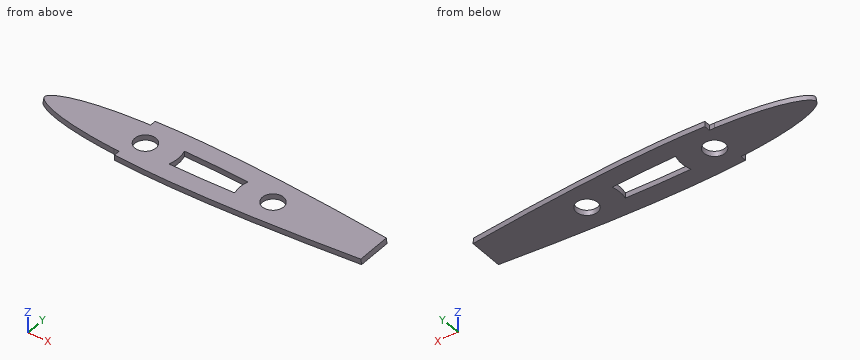
```python
from build123d import *

# Parameters (mm, degrees)
BOSS_EXTRUDE1_DEPTH     = 3.175
SKETCH2_R               = 6.35
CUT_EXTRUDE1_DEPTH      = 3.175
CUT_EXTRUDE2_DEPTH      = 17.98531302
CUT_EXTRUDE2_DEPTH_BACK = 17.98531302
CUT_EXTRUDE3_DEPTH      = 7.62


with BuildPart() as part:
    # Sketch1 → Boss-Extrude1 (new body)
    with BuildSketch(Plane.XY):
        with BuildLine():
            add(Edge.make_bspline(
                [(283.0068, 0.356588568), (282.901747419, 0.44462405), (282.222988768, 0.361501496), (281.014292834, 0.701750535), (278.797705315, 0.912055534), (275.811625252, 1.363395917), (271.96510687, 1.867061556), (267.326448481, 2.487806401), (261.907718596, 3.189499382), (255.748156548, 3.970743632), (248.883761402, 4.817852882), (241.357474346, 5.719362844), (233.215556988, 6.664092103), (224.508147533, 7.639178426), (215.288960535, 8.632716794), (205.614900546, 9.632367333), (195.545587828, 10.625227013), (185.143130495, 11.597359066), (174.471591387, 12.536001404), (163.596880752, 13.425461607), (152.585818931, 14.251236992), (141.506392817, 14.997996378), (130.426867175, 15.650125673), (119.415450083, 16.19114965), (108.540147703, 16.606641404), (97.867696152, 16.883046032), (87.464049003, 17.006862886), (77.393132365, 16.968265808), (67.717036062, 16.75979946), (58.495320886, 16.376179449), (49.784748261, 15.816402284), (41.638853683, 15.082152298), (34.107484228, 14.179164014), (27.236546007, 13.115120527), (21.067675242, 11.901134861), (15.637028536, 10.550933877), (10.975465177, 9.077683717), (7.106668967, 7.49510566), (4.042977604, 5.813906592), (1.789105378, 4.030768344), (0.345518556, 2.10255275), (-0.161023932, 0), (0.345518556, -2.10255275), (1.789105378, -4.030768344), (4.042977604, -5.813906592), (7.106668967, -7.49510566), (10.975465177, -9.077683717), (15.637028536, -10.550933877), (21.067675242, -11.901134861), (27.236546007, -13.115120527), (34.107484228, -14.179164014), (41.638853683, -15.082152298), (49.784748261, -15.816402284), (58.495320886, -16.376179449), (67.717036062, -16.75979946), (77.393132365, -16.968265808), (87.464049003, -17.006862886), (97.867696152, -16.883046032), (108.540147703, -16.606641404), (119.415450083, -16.19114965), (130.426867175, -15.650125673), (141.506392817, -14.997996378), (152.585818931, -14.251236992), (163.596880752, -13.425461607), (174.471591387, -12.536001404), (185.143130495, -11.597359066), (195.545587828, -10.625227013), (205.614900546, -9.632367333), (215.288960535, -8.632716794), (224.508147533, -7.639178426), (233.215556988, -6.664092103), (241.357474346, -5.719362844), (248.883761402, -4.817852882), (255.748156548, -3.970743632), (261.907718596, -3.189499382), (267.326448481, -2.487806401), (271.96510687, -1.867061556), (275.811625252, -1.363395917), (278.797705315, -0.912055534), (281.014292834, -0.701750535), (282.222988768, -0.361501496), (283.176929529, -0.478323569), (283.176929529, 0.214017725), (283.0068, 0.356588568)],
                knots=[0, 0, 0, 0, 0.000762215, 0.003044706, 0.006832246, 0.012101176, 0.018817536, 0.026939455, 0.036414848, 0.047184628, 0.059180413, 0.072327874, 0.086544061, 0.10174058, 0.117823336, 0.134691452, 0.152240154, 0.17036129, 0.188941008, 0.207865435, 0.227016078, 0.246275696, 0.265524943, 0.284644966, 0.303520118, 0.322034575, 0.340078353, 0.357542593, 0.374325482, 0.390329891, 0.40546389, 0.419643801, 0.432793371, 0.444843817, 0.455737921, 0.465428653, 0.47388632, 0.481101634, 0.487101684, 0.491975368, 0.495930678, 0.499382808, 0.502834938, 0.506790248, 0.511663932, 0.517663982, 0.524879296, 0.533336963, 0.543027695, 0.553921799, 0.565972245, 0.579121815, 0.593301726, 0.608435725, 0.624440134, 0.641223023, 0.658687263, 0.676731041, 0.695245498, 0.71412065, 0.733240673, 0.75248992, 0.771749538, 0.790900181, 0.809824608, 0.828404326, 0.846525462, 0.864074164, 0.88094228, 0.897025036, 0.912221555, 0.926437743, 0.939585203, 0.951580988, 0.962350768, 0.971826162, 0.979948081, 0.986664441, 0.991933371, 0.99572091, 0.998003402, 0.998765616, 1, 1, 1, 1], degree=3))
        make_face()
    extrude(amount=BOSS_EXTRUDE1_DEPTH)

    # Sketch2 → Cut-Extrude1 (cut)
    with BuildSketch(Plane.XY.offset(3.175)):
        with Locations((63.5, 0)):
            Circle(SKETCH2_R)
        with Locations((139.7, 0)):
            Circle(SKETCH2_R)
    extrude(amount=-CUT_EXTRUDE1_DEPTH, mode=Mode.SUBTRACT)

    # Sketch3 → Cut-Extrude2 (cut, two sides)
    with BuildSketch(Plane(origin=(0, 0, 0), x_dir=(1, 0, 0), z_dir=(0, 1, 0))) as cut_extrude2_sk:
        Polygon((280.502264678, 570.685147201), (200.220132014, 0), (199.773483328, -3.175), (283.134397147, -3.175), (283.134397147, 0), (283.134397147, 576.304397051), (-760.640477334, 1065.222635252), (-763.272609802, 1059.603385401), align=None)
    extrude(amount=CUT_EXTRUDE2_DEPTH, mode=Mode.SUBTRACT)
    extrude(cut_extrude2_sk.sketch, amount=-CUT_EXTRUDE2_DEPTH_BACK, mode=Mode.SUBTRACT)

    # Sketch5 → Cut-Loft1 section 0
    with BuildSketch(Plane.XY.offset(3.175)):
        with BuildLine():
            Line((57.15, -15.840717611), (57.15, -12.517848774))
            Line((57.15, -12.517848774), (54.102, -12.517848774))
            add(Edge.make_bspline(
                [(54.102, 12.517848774), (52.905073826, 12.446922239), (50.510877245, 12.29292233), (46.923042309, 12.02249839), (43.342906141, 11.709637993), (39.772343425, 11.350207554), (36.212958119, 10.940125109), (32.668672918, 10.473083309), (29.140579279, 9.942416236), (26.221744689, 9.439792705), (23.899631399, 8.996334016), (22.168124881, 8.641223297), (20.447130555, 8.261260302), (18.73921392, 7.85440932), (17.04583843, 7.418483842), (15.37131979, 6.950314461), (13.720374707, 6.446953018), (12.099093951, 5.903590986), (10.516736009, 5.316840777), (8.982942702, 4.676356823), (7.515425701, 3.975597981), (6.148367378, 3.214391725), (5.132435214, 2.525362189), (4.436328841, 1.942644965), (3.99449908, 1.50088383), (3.639558845, 1.055711416), (3.418173473, 0.67028204), (3.294529971, 0.303832168), (3.258254336, 8.98e-07), (3.294531501, -0.303834398), (3.41817022, -0.670279004), (3.63956519, -1.05571658), (3.994486701, -1.500874192), (4.436322379, -1.942640233), (5.13276687, -2.525613649), (6.148175252, -3.21424607), (7.515525046, -3.97567324), (8.982885795, -4.676313816), (10.516775422, -5.316870372), (12.099068229, -5.90357211), (13.720394844, -6.446967156), (15.371289631, -6.95029465), (17.045828606, -7.418477981), (18.739219111, -7.854412516), (20.44713727, -8.261264475), (22.168119663, -8.641219802), (23.899622625, -8.996332253), (26.221845214, -9.439810116), (29.140506404, -9.942404258), (32.668709943, -10.473088914), (36.212941173, -10.940123046), (39.772346311, -11.350206942), (43.342914131, -11.709640819), (46.923012021, -12.0224901), (50.510859023, -12.292917903), (52.905073826, -12.446922239), (54.102, -12.517848774)],
                knots=[0, 0, 0, 0, 0.03125, 0.0625, 0.09375, 0.125, 0.15625, 0.1875, 0.21875, 0.25, 0.265625, 0.28125, 0.296875, 0.3125, 0.328125, 0.34375, 0.359375, 0.375, 0.390625, 0.40625, 0.421875, 0.4375, 0.453125, 0.4609375, 0.46875, 0.4765625, 0.484375, 0.4921875, 0.5, 0.5078125, 0.515625, 0.5234375, 0.53125, 0.5390625, 0.546875, 0.5625, 0.578125, 0.59375, 0.609375, 0.625, 0.640625, 0.65625, 0.671875, 0.6875, 0.703125, 0.71875, 0.734375, 0.75, 0.78125, 0.8125, 0.84375, 0.875, 0.90625, 0.9375, 0.96875, 1, 1, 1, 1], degree=3))
            Line((54.102, 12.517848774), (57.15, 12.517848774))
            Line((57.15, 12.517848774), (57.15, 15.840717611))
            Line((57.15, 15.840717611), (57.15, 24.528656823))
            Line((57.15, 24.528656823), (-13.660315185, 32.196838039))
            Line((-13.660315185, 32.196838039), (4.751362513, -35.926369443))
            Line((4.751362513, -35.926369443), (57.15, -29.012871964))
            Line((57.15, -29.012871964), (57.15, -15.840717611))
        make_face()
    # Sketch4 → Cut-Loft1 section 1
    with BuildSketch(Plane(origin=(0, 0, 0), x_dir=(-1, 0, 0), z_dir=(0, 0, -1))):
        with BuildLine():
            Line((-57.15, -15.931097341), (-57.15, -12.614401813))
            Line((-57.15, -12.614401813), (-54.102, -12.614401813))
            add(Edge.make_bspline(
                [(-54.102, 12.614401813), (-52.892966304, 12.543650374), (-50.474562395, 12.389900929), (-46.850429349, 12.119518431), (-43.233994008, 11.80632974), (-39.627106768, 11.446155851), (-36.031309682, 11.034861155), (-32.450571185, 10.566087473), (-28.885974607, 10.033109549), (-25.936699002, 9.527992325), (-23.590171059, 9.082138578), (-21.840349809, 8.725010585), (-20.101018277, 8.342781179), (-18.374759552, 7.933393598), (-16.663038707, 7.494638099), (-14.970151675, 7.023265253), (-13.3008012, 6.516250081), (-11.661107617, 5.968693544), (-10.06037111, 5.377118947), (-8.508330893, 4.731019213), (-7.022897298, 4.023737888), (-5.63853584, 3.25470078), (-4.609088563, 2.55765795), (-3.903506054, 1.967798123), (-3.455598612, 1.52050909), (-3.095749955, 1.069692125), (-2.871302388, 0.679325256), (-2.745924545, 0.30796261), (-2.7091298, 9.1e-07), (-2.745926097, -0.307964873), (-2.871299087, -0.679322175), (-3.095756394, -1.069697364), (-3.455586055, -1.520499314), (-3.903499495, -1.967793321), (-4.609425021, -2.557913052), (-5.638340949, -3.254553026), (-7.022998045, -4.023814214), (-8.50827323, -4.730975626), (-10.060410962, -5.377148887), (-11.661081805, -5.968674575), (-13.300821123, -6.516264103), (-14.970122445, -7.02324602), (-16.6630295, -7.494632633), (-18.374764393, -7.933396571), (-20.10102481, -8.342785237), (-21.840344745, -8.725007186), (-23.590162295, -9.082136874), (-25.936800786, -9.528009858), (-28.88590077, -10.033097475), (-32.450608778, -10.56609314), (-36.031292313, -11.034859029), (-39.627110143, -11.446155342), (-43.234001329, -11.806332406), (-46.850400529, -12.119510514), (-50.474544843, -12.389896679), (-52.892966304, -12.543650374), (-54.102, -12.614401813)],
                knots=[0, 0, 0, 0, 0.03125, 0.0625, 0.09375, 0.125, 0.15625, 0.1875, 0.21875, 0.25, 0.265625, 0.28125, 0.296875, 0.3125, 0.328125, 0.34375, 0.359375, 0.375, 0.390625, 0.40625, 0.421875, 0.4375, 0.453125, 0.4609375, 0.46875, 0.4765625, 0.484375, 0.4921875, 0.5, 0.5078125, 0.515625, 0.5234375, 0.53125, 0.5390625, 0.546875, 0.5625, 0.578125, 0.59375, 0.609375, 0.625, 0.640625, 0.65625, 0.671875, 0.6875, 0.703125, 0.71875, 0.734375, 0.75, 0.78125, 0.8125, 0.84375, 0.875, 0.90625, 0.9375, 0.96875, 1, 1, 1, 1], degree=3))
            Line((-54.102, 12.614401813), (-57.15, 12.614401813))
            Line((-57.15, 12.614401813), (-57.15, 15.931097341))
            Line((-57.15, 15.931097341), (-57.15, 23.768946795))
            Line((-57.15, 23.768946795), (16.290986713, 29.461293478))
            Line((16.290986713, 29.461293478), (3.107394198, -36.097931887))
            Line((3.107394198, -36.097931887), (-57.15, -26.910981695))
            Line((-57.15, -26.910981695), (-57.15, -15.931097341))
        make_face()
    loft(mode=Mode.SUBTRACT)

    # Sketch6 → Cut-Extrude3 (cut)
    with BuildSketch(Plane(origin=(0, 0, 0), x_dir=(-1, 0, 0), z_dir=(0, 0, -1))):
        with BuildLine():
            ThreePointArc((-120.7436607, -5.30626284), (-120.015, 0), (-120.7436607, 5.30626284))
            add(Edge.make_bspline(
                [(-120.7436607, 5.30626284), (-116.113978677, 5.516834405), (-111.486849996, 5.695579464), (-101.374008891, 6.004242594), (-95.890716435, 6.118585943), (-87.671447186, 6.189682577), (-84.92815734, 6.19667575), (-82.188251061, 6.184536948)],
                knots=[0.519741838, 0.519741838, 0.519741838, 0.519741838, 0.625, 0.625, 0.75, 0.75, 0.812699407, 0.812699407, 0.812699407, 0.812699407], degree=3))
            ThreePointArc((-82.188251061, 6.184536948), (-83.185, 0), (-82.188251061, -6.184536948))
            add(Edge.make_bspline(
                [(-82.188251061, -6.184536948), (-84.92815734, -6.19667575), (-87.671447186, -6.189682577), (-95.890716436, -6.118585943), (-101.374008891, -6.004242594), (-111.486849996, -5.695579464), (-116.113978677, -5.516834405), (-120.7436607, -5.30626284)],
                knots=[0.187300593, 0.187300593, 0.187300593, 0.187300593, 0.25, 0.25, 0.375, 0.375, 0.480258162, 0.480258162, 0.480258162, 0.480258162], degree=3))
        make_face()
    extrude(amount=-CUT_EXTRUDE3_DEPTH, mode=Mode.SUBTRACT)


solid = part.part
```
Build history of the part. All positions in model axes, mm. Round coordinates to 2 decimals unless told otherwise and drop trailing zeros.
1) Drill centre lines: probe 1 along X at (y, z) = (-2, 0.9); probe 2 along X at (y, z) = (-3, 3); probe 3 along Y at (x, z) = (114, 2.05). Where is each one in solid material? Low to high.
2) Band-saw the part on A-A, the plane y = 0. Give the number of separate pieces and of enclosed holes in the cut face, and give its area (3 significant figures).
3) Pin check, flat tip, straight feed: pin 1 (1 mm diameter, centred on x = 77.5, z = 3, fed in from -Y). Stop position of the tip, or through.
Ans:
1. probe 1: x = 4.11 to 57.47, 69.53 to 83.08, 120.12 to 133.67, 145.73 to 200.09
1. probe 2: x = 5.82 to 57.9, 69.1 to 82.96, 120.24 to 134.1, 145.3 to 199.8
1. probe 3: y = -16.39 to -5.59, 5.59 to 16.39
2. separate pieces: 4
2. enclosed holes: 0
2. area: 428 mm2
3. pin 1: stops at y = -16.95
